Work out the finished part from the listing and answer in its coordinate system (mm). Face numbers are marked on the shaded views. Round coordinates to 2 decimals unless told otherwise and drop trailing zeros. Order: outer loops, then holes, each group sorted by start corner. A loop starts at its lowest first (then second) coordinate and runs counter-clockwise, first axis right, second up. Notation, with made-up numbers: M -1.75,19 L 57.25,19 A27 ccw 57.25,48 Z; hole C 56,68 d5. An arc over 180 degrees is marked long. Return JSON: item names as keys, results as strings.
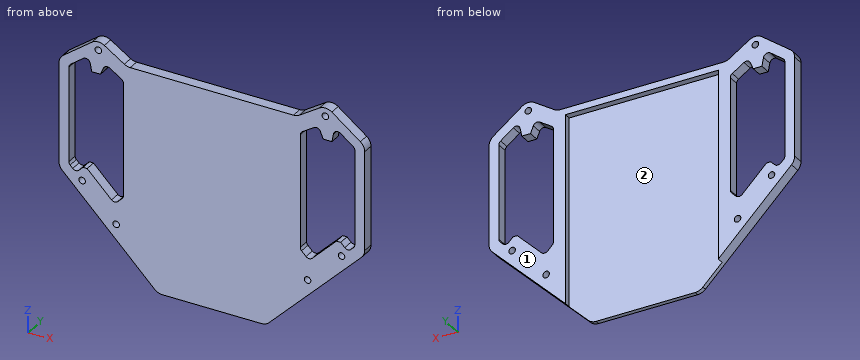
from build123d import *

# Parameters (mm, degrees)
SKETCH1_R            = 1.5
BOSS_EXTRUDE1_DEPTH  = 5
FILLET1_R            = 2
FILLET1_OF_MIRROR1_R = 2
SKETCH2_W            = 70
SKETCH2_H            = 97
CUT_EXTRUDE1_DEPTH   = 3
FILLET2_R            = 5


with BuildPart() as part:
    # Sketch1 → Boss-Extrude1 (new body)
    with BuildSketch(Plane(origin=(0, 0, 0), x_dir=(1, 0, 0), z_dir=(0, 1, 0))):
        Polygon((-52.164149312, -38.645247828), (-70, -25.247940817), (-70, 24.752308679), (-24.752308679, 70), (0, 70), (0, -30), (-38.851635079, -30), align=None)
        with Locations((-43.840620434, 43.840620434)):
            Circle(SKETCH1_R, mode=Mode.SUBTRACT)
        with Locations((-51.997575213, -33.767620171)):
            Circle(SKETCH1_R, mode=Mode.SUBTRACT)
        with Locations((-59.39696962, 28.284271247)):
            Circle(SKETCH1_R, mode=Mode.SUBTRACT)
        Polygon((-59.003765723, 22.1), (-57.095959493, 22.1), (-44.547727215, 34.648232278), (-40.5, 30.600505063), (-40.5, -23), (-48.796166422, -28.387593469), (-51, -23), (-55, -23), (-56.33662338, -29.883022962), (-65.5, -23), (-65.5, 22.181240867), (-62.292503295, 25.388737572), align=None, mode=Mode.SUBTRACT)
    boss_extrude1 = extrude(amount=BOSS_EXTRUDE1_DEPTH)

    # Fillet1
    fillet1_edges = [part.edges().sort_by_distance(p)[0] for p in [
        (-44.547727215, 2.5, -34.648232278),
        (-62.292503295, 2.5, -25.388737572),
        (-65.5, 2.5, -22.181240867),
        (-65.5, 2.5, 23),
        (-56.33662338, 2.5, 29.883022962),
        (-48.796166422, 2.5, 28.387593469),
        (-40.5, 2.5, 23),
        (-40.5, 2.5, -30.600505063),
    ]]
    fillet(fillet1_edges, radius=FILLET1_R)

    # Mirror1: Boss-Extrude1 across plane
    add(boss_extrude1.mirror(Plane(origin=(0, 5, 30), x_dir=(0, 0, 1), z_dir=(-1, 0, 0))))

    # Fillet1 of Mirror1
    fillet1_of_mirror1_edges = [part.edges().sort_by_distance(p)[0] for p in [
        (44.547727215, 2.5, -34.648232278),
        (62.292503295, 2.5, -25.388737572),
        (65.5, 2.5, -22.181240867),
        (65.5, 2.5, 23),
        (56.33662338, 2.5, 29.883022962),
        (48.796166422, 2.5, 28.387593469),
        (40.5, 2.5, 23),
        (40.5, 2.5, -30.600505063),
    ]]
    fillet(fillet1_of_mirror1_edges, radius=FILLET1_OF_MIRROR1_R)

    # Sketch2 → Cut-Extrude1 (cut)
    with BuildSketch(Plane(origin=(0, 5, 0), x_dir=(1, 0, 0), z_dir=(0, 1, 0))):
        with Locations((0, 21.5)):
            Rectangle(SKETCH2_W, SKETCH2_H)
    extrude(amount=-CUT_EXTRUDE1_DEPTH, mode=Mode.SUBTRACT)

    # Fillet2
    fillet2_edges = [part.edges().sort_by_distance(p)[0] for p in [
        (-70, 2.5, -24.752308679),
        (70, 2.5, 25.247940817),
        (70, 2.5, -24.752308679),
        (38.851635079, 2.5, 30),
        (-38.851635079, 2.5, 30),
        (52.164149312, 2.5, 38.645247828),
        (-52.164149312, 2.5, 38.645247828),
        (-70, 2.5, 25.247940817),
        (24.752308679, 1, -70),
        (-24.752308679, 1, -70),
    ]]
    fillet(fillet2_edges, radius=FILLET2_R)


solid = part.part
Item 1: Find section B-B (x = -11). Determine the outline of the cut face in (y, z), plus the area to 3 significant figures.
Output:
{"outline": "M 0,-70 L 2,-70 L 2,27 L 5,27 L 5,30 L 0,30 Z", "area": "209 mm^2"}
Item 2: Find section D-D (y = 1.15). State how many separate pieces and enclosed holes the cut face has, plus the area to 3 significant figures.
Output:
{"separate pieces": "1", "enclosed holes": "8", "area": "9,450 mm^2"}
Item 3: Each of these flat-tipped pins is pushed along its axis until it touches: pin 1 (5 mm diameter, centred on x = -22, z = -11, fed in from -Y); pin 2 (1.8 mm diameter, centred on x = -52, z = 33.77, fed in from -Y); pin 3 (2 mm diameter, centred on x = 53, y = 1.5, fed in from -Z); pin 4 (2 mm diameter, centred on x = -58, y = 2.5, fed in from +Z). Where does it stop, or does it pass through?
Output:
{"pin 1": "stops at y = 0", "pin 2": "passes through", "pin 3": "stops at z = -42.75", "pin 4": "stops at z = 35.01"}
Item 4: Find section A-A (z = -10.5). Determine the outline of the cut face in (x, y).
Output:
{"outline": "M -70,0 L -65.5,0 L -65.5,5 L -70,5 Z; M -40.5,0 L 40.5,0 L 40.5,5 L 35,5 L 35,2 L -35,2 L -35,5 L -40.5,5 Z; M 65.5,0 L 70,0 L 70,5 L 65.5,5 Z"}
Item 5: Find section C-C (z = -56). Determine the outline of the cut face in (x, y).
Output:
{"outline": "M -38.75,0 L 38.75,0 L 38.75,5 L 35,5 L 35,2 L -35,2 L -35,5 L -38.75,5 Z"}
Item 6: The mould has two halves that part along X. Classify the marked faces 1 and 2: pulls with the +X half, pulls with the -X half, needs draft (parallel to the pull), parting line crosses it, or undercut.
Output:
{"face 1": "needs draft", "face 2": "undercut"}
Item 7: Consider line 1 along X through (y, z) = (2.35, 3.5); line 2 along X through (y, z) = (1.2, -12.5); line 3 along Z through (x, y) = (60.5, 3.1). Determine where each line is inside the solid, lowest interval first. Write a range as [from, to].
Output:
{"line 1": "x = [-70, -65.5], [-40.5, -35], [35, 40.5], [65.5, 70]", "line 2": "x = [-70, -65.5], [-40.5, 40.5], [65.5, 70]", "line 3": "z = [-34.25, -29.3], [-27.27, -23.6], [26.76, 32.38]"}
